For this review, take the finished solid that the model builds, in its own axes (mm). A direction names the side the tool comes from. Round coordinates to 2 decimals unless told otherwise and drop trailing zeros. Write each loop counter-clockwise with the first axis right and the second up, starting at its lowest first coordinate (ties: lowest second). Pieces come first, ordered by that corner, then holes. Notation, with made-up numbers: M 55,28 L 70,28 A5 cw 70,34 Z; hole C 34.25,66.5 d3. An arc over 180 degrees is marked long. Use one line per item in the form item = value. Start each with the question number.
Item 1: Add section C-C (y = -2.5). Count the separate pieces of the cut face and the enclosed holes in it, and give its area (3 significant figures).
Item 2: Add section A-A (z = 114.3). State the section outline as (x, y) points (3 decimals).
Item 3: Draft analysis for pull direction Z (two halves, no side actions). For faces 4 (the flat face through (41.275, -3, 94)), 5 (the flat face through (56, -6.35, 89)), 6 (the cylindrical face through (74.098, -3.219, 2.835)), state which applies: released by +Z, released by -Z, zero draft, split by the parting line, or undercut.
Item 4: Add section B-B (z = 53). State the section outline as (x, y) points (3 decimals), and give its area (3 significant figures).
Item 5: For faces 1 (the flat face through (41.275, -3, 55)), 2 (the flat face through (14, -3, -12.702)), 3 (the flat face through (20, -3, 0)), list the 3-axis set-ups (+Z, -Z, +X, -X, +Y, -Y) from which the entire face can be reached by the end or side of a thin tool; tool diameter is ignored.
Item 6: For P1, Ø3, axis at y = -3, z = 31.5, coming from the -X side; P2, Ø1.5, axis at x = 45.5, y = -3, coming from the -Z side (3 decimals); P3, Ø2, axis at y = -4, z = 16, coming from the +X side, all flat-tipped, find the tip position at first contact; note any pin that passes through.
Item 7: For line 1 (X direction, y = -2.75, z = 47); line 2 (X direction, y = -4, z = 78); line 3 (X direction, y = -3.75, z = 80.5), list the stretches that pass through material, from the lowest coordinate up. Write a range as [from, to].
from build123d import *

# Parameters (mm, degrees)
F0_R     = 19.685
F1_DEPTH = 6.35
F2_R     = 2.54
F3_R     = 12.7
F5_DEPTH = 6.351


with BuildPart() as f1:
    # F0 (on Front) → F1 (new body)
    with BuildSketch(Plane.XZ):
        with BuildLine():
            Line((0, -6.351505), (0, 0))
            Line((0, 0), (41.275, 0))
            Line((41.275, 0), (41.275, 9.525))
            Line((41.275, 9.525), (53.975, 9.525))
            Line((53.975, 9.525), (53.975, 0))
            Line((53.975, 0), (76.2, 0))
            Line((76.2, 0), (100.622425, 105.724714))
            ThreePointArc((100.622425, 105.724714), (74.146687, 150.88221), (27.573491, 126.984477))
            Line((27.573491, 126.984477), (-12.608211, 13.177002))
            Line((-12.608211, 13.177002), (-12.608211, -12.701505))
            Line((-12.608211, -12.701505), (31.75, -12.701505))
            Line((31.75, -12.701505), (31.75, -6.351505))
            Line((31.75, -6.351505), (0, -6.351505))
        make_face()
        with Locations((63.5, 114.3)):
            Circle(F0_R, mode=Mode.SUBTRACT)
    extrude(amount=F1_DEPTH)

    # F2
    f2_edges = [f1.edges().sort_by_distance(p)[0] for p in [
        (31.75, -3.175, -6.351505),
        (31.75, -3.175, -12.701505),
        (41.275, -3.175, 9.525),
        (53.975, -3.175, 9.525),
    ]]
    fillet(f2_edges, radius=F2_R)

    # F3
    f3_edges = [f1.edges().sort_by_distance(p)[0] for p in [
        (-12.608211, -3.175, -12.701505),
        (-12.608211, -3.175, 13.177002),
        (76.2, -3.175, 0),
    ]]
    fillet(f3_edges, radius=F3_R)

    # F4 (on Front) → F5 (cut, through all)
    with BuildSketch(Plane.XZ):
        with BuildLine():
            ThreePointArc((41.275, 95.345489), (36.780001, 102.498908), (34.520263, 110.639546))
            Line((34.520263, 110.639546), (32.346901, 111.894337))
            Line((32.346901, 111.894337), (23.745077, 87.531209))
            Line((23.745077, 87.531209), (28.575, 84.742652))
            Line((28.575, 84.742652), (41.275, 92.075))
            Line((41.275, 92.075), (41.275, 95.345489))
        make_face()
        Polygon((-3.175, 11.284914), (-3.796368, 9.525), (-3.175, 9.525), align=None)
        with BuildLine():
            Line((63.229602, 9.525), (66.099263, 9.525))
            ThreePointArc((66.099263, 9.525), (68.075591, 10.215095), (69.192798, 11.985393))
            Line((69.192798, 11.985393), (72.117945, 24.648357))
            Line((72.117945, 24.648357), (60.325, 17.839697))
            Line((60.325, 17.839697), (60.325, 15.141723))
            ThreePointArc((60.325, 15.141723), (62.151813, 12.527035), (63.229602, 9.525))
        make_face()
        with BuildLine():
            Line((49.098523, 19.05), (51.435, 19.05))
            ThreePointArc((51.435, 19.05), (51.933052, 19.039716), (52.430256, 19.00888))
            Line((52.430256, 19.00888), (63.5, 25.4))
            Line((63.5, 25.4), (63.5, 40.064697))
            Line((63.5, 40.064697), (50.8, 47.397045))
            Line((50.8, 47.397045), (38.1, 40.064697))
            Line((38.1, 40.064697), (38.1, 25.4))
            Line((38.1, 25.4), (49.098523, 19.05))
        make_face()
        with BuildLine():
            Line((15.875, 9.525), (32.020398, 9.525))
            ThreePointArc((32.020398, 9.525), (34.885752, 15.098738), (40.160436, 18.483191))
            Line((40.160436, 18.483191), (28.575, 25.172045))
            Line((28.575, 25.172045), (15.875, 17.839697))
            Line((15.875, 17.839697), (15.875, 9.525))
        make_face()
        Polygon((19.05, 40.064697), (9.028931, 45.850364), (0.427107, 21.487236), (6.35, 18.067652), (19.05, 25.4), align=None)
        Polygon((19.05, 69.85), (19.05, 74.233246), (17.106185, 68.727738), align=None)
        with BuildLine():
            Line((63.5, 84.514697), (62.472217, 85.108087))
            ThreePointArc((62.472217, 85.108087), (54.623617, 86.471347), (47.435202, 89.904378))
            Line((47.435202, 89.904378), (38.1, 84.514697))
            Line((38.1, 84.514697), (38.1, 69.85))
            Line((38.1, 69.85), (50.8, 62.517652))
            Line((50.8, 62.517652), (63.5, 69.85))
            Line((63.5, 69.85), (63.5, 84.514697))
        make_face()
        Polygon((86.469863, 86.777831), (82.55, 84.514697), (82.55, 69.85), (82.55841, 69.845145), align=None)
        Polygon((15.875, 62.289697), (15.875, 47.625), (28.575, 40.292652), (41.275, 47.625), (41.275, 62.289697), (28.575, 69.622045), align=None)
        Polygon((60.325, 62.289697), (60.325, 47.625), (73.025, 40.292652), (76.148332, 42.095908), (81.391103, 64.791873), (73.025, 69.622045), align=None)
        with BuildLine():
            Line((70.8124, 86.020097), (73.025, 84.742652))
            Line((73.025, 84.742652), (85.725, 92.075))
            Line((85.725, 92.075), (85.725, 95.345489))
            ThreePointArc((85.725, 95.345489), (78.98726, 89.533715), (70.8124, 86.020097))
        make_face()
    extrude(amount=F5_DEPTH, mode=Mode.SUBTRACT)


solid = f1.part
Calculated:
q1.separate_pieces = 1
q1.enclosed_holes = 13
q1.area = 8,060 mm^2
q2.outline = M 23.095,-6.35 L 43.815,-6.35 L 43.815,0 L 23.095,0 Z; M 83.185,-6.35 L 101.6,-6.35 L 101.6,0 L 83.185,0 Z
q3.face_4 = undercut
q3.face_5 = zero draft
q3.face_6 = released by -Z
q4.outline = M 1.452,-6.35 L 15.875,-6.35 L 15.875,0 L 1.452,0 Z; M 41.275,-6.35 L 60.325,-6.35 L 60.325,0 L 41.275,0 Z; M 78.667,-6.35 L 88.443,-6.35 L 88.443,0 L 78.667,0 Z
q4.area = 275 mm^2
q5.face_1 = +Y, -Y
q5.face_2 = -Z, +X, -X, +Y, -Y
q5.face_3 = +X, +Y, -Y
q6.P1 = -6.67
q6.P2 = 9.525
q6.P3 = 80.13
q7.line_1 = [-0.67, 16.96], [40.19, 50.11], [51.49, 61.41], [77.28, 87.06]
q7.line_2 = [10.28, 38.1], [63.5, 82.55], [84.44, 94.22]
q7.line_3 = [11.16, 38.1], [63.5, 82.55], [85.02, 94.8]
